The listing builds one solid part. Answer for the finished solid, in the listing's coordinates (mm). Face numbers are marked on the shaded views. A direction names the side the tool comes from. Round coordinates to 2 decimals unless told otherwise and drop trailing zeros. Write each loop counter-clockwise with the first axis right and the second up, starting at its lowest first coordinate (ties: lowest second). Pieces come first, ordered by that corner, then holes. Notation, with made-up numbers: (29, 61) - (41, 61) arc R21 ccw to (41, 66) - close; hole circle Ø5 at (10, 86). An arc over 180 degrees is marked (long way). Return JSON: item names as keys, results as strings. Group by question number.
(1) Section C-C, the plane z = 21.5 is taken. Write down the section's boundary in (x, y).
(2) Find the intervals of material crossed by line 1 along X through (y, z) = (-15.25, 28); line 2 along Z through (x, y) = (29, -16.5); line 3 along Y through (x, z) = (16.5, 14), in increasing order. Write a range as [from, to].
(3) Section B-B, the plane y = -11 is taken. Write down the section's boundary in (x, z).
(4) Which of the six approach directions +Z, -Z, +X, -X, +Y, -Y give full straight-line access (tool end or side, diameter ignored) to the marked faces 1 and 2?
(5) Section A-A, the plane x = 30 is taken. Write down the section's boundary in (y, z).
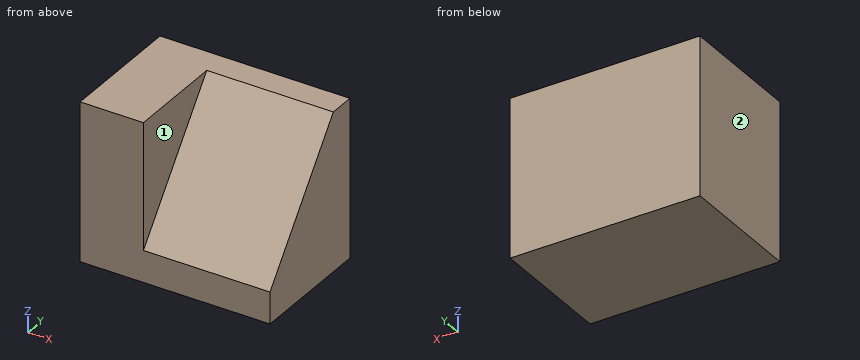
```python
from build123d import *

# Parameters (mm, degrees)
F0_W     = 25.4
F0_H     = 31.75
F1_DEPTH = 12.7
F3_DEPTH = 25.4


with BuildPart() as f1:
    # F0 (on Right) → F1 (new body)
    with BuildSketch(Plane.YZ):
        with Locations((-12.7, 15.875)):
            Rectangle(F0_W, F0_H)
    extrude(amount=F1_DEPTH)

    # F2 (on face) → F3 (join)
    with BuildSketch(Plane.YZ.offset(12.7)):
        Polygon((0, 0), (0, 31.75), (-5.256133, 31.75), (-25.4, 6.35), (-25.4, 0), align=None)
    extrude(amount=F3_DEPTH)


solid = f1.part
```
Working result:
{
 "1": {"outline": "(0, -25.4) - (12.7, -25.4) - (12.7, -13.39) - (38.1, -13.39) - (38.1, 0) - (0, 0) - close"},
 "2": {"line 1": "x = [0, 12.7]", "line 2": "z = [0, 17.57]", "line 3": "y = [-19.33, 0]"},
 "3": {"outline": "(0, 0) - (38.1, 0) - (38.1, 24.51) - (12.7, 24.51) - (12.7, 31.75) - (0, 31.75) - close"},
 "4": {"face 1": "+Z, +X, -Y", "face 2": "+Z, -Z, -X, +Y, -Y"},
 "5": {"outline": "(-25.4, 0) - (0, 0) - (0, 31.75) - (-5.26, 31.75) - (-25.4, 6.35) - close"}
}
